Read the model definition and answer for the solid it produces. Units are mm, in the model's axes. A direction names the side the tool comes from. Round coordinates to 2 decimals unless told otherwise and drop trailing zeros. Write each loop counter-clockwise with the first axis right and the second up, starting at its lowest first coordinate (ties: lowest second). Pieces come first, ordered by that corner, then holes. Notation, with made-up numbers: (20, 70.25) -> (54, 70.25) arc R28 ccw to (54, 91.25) -> close; hole circle Ø8 at (-19.5, -8.5). An arc over 180 degrees is marked (long way). Return JSON: item names as keys, results as strings.
from build123d import *

# Parameters (mm, degrees)
SKETCH_1_R          = 7
SKETCH_1_R_2        = 1.5
EXTRUDE_1_DEPTH     = 14
FILLET_2_R          = 1
FILLET_4_R          = 2
FILLET_5_R          = 1
CUT_EXTRUDE_1_DEPTH = 10
FILLET_6_R          = 1
SKETCH_4_R          = 43
SKETCH_4_W          = 56
SKETCH_4_H          = 56
CUT_EXTRUDE_2_DEPTH = 2


with BuildPart() as part:
    # 草图1 → 凸台-拉伸1 (new body)
    # profile 1 of 3: a face of its own
    with BuildSketch(Plane.XY):
        with BuildLine():
            Line((-2.5, 7), (-20, 7))
            ThreePointArc((-20, 7), (-15.050252532, 4.949747468), (-13, 0))
            ThreePointArc((-13, 0), (-15.050252532, -4.949747468), (-20, -7))
            Line((-20, -7), (0, -7))
            ThreePointArc((0, -7), (-4.949747468, 4.949747468), (7, 0))
            Line((7, 0), (7, 4))
            Line((7, 4), (12, 4))
            Line((12, 4), (12, 5))
            Line((12, 5), (6.5, 9))
            Line((6.5, 9), (3.5, 9))
            Line((3.5, 9), (3.5, 26))
            Line((3.5, 26), (-2.5, 26))
            Line((-2.5, 26), (-2.5, 7))
        make_face()
    # profile 2 of 3: a face of its own
    with BuildSketch(Plane.XY):
        Circle(SKETCH_1_R)
        Circle(SKETCH_1_R_2, mode=Mode.SUBTRACT)
    # profile 3 of 3: a face of its own
    with BuildSketch(Plane.XY):
        with Locations((-20, 0)):
            Circle(SKETCH_1_R)
        with Locations((-20, 0)):
            Circle(SKETCH_1_R_2, mode=Mode.SUBTRACT)
    extrude(amount=EXTRUDE_1_DEPTH)

    # 圆角2
    fillet_2_edges = [part.edges().sort_by_distance(p)[0] for p in [
        (-2.5, 7, 7),
        (7, 4, 7),
    ]]
    fillet(fillet_2_edges, radius=FILLET_2_R)

    # 圆角4
    fillet_4_edges = [part.edges().sort_by_distance(p)[0] for p in [
        (6.5, 9, 7),
    ]]
    fillet(fillet_4_edges, radius=FILLET_4_R)

    # 圆角5
    fillet_5_edges = [part.edges().sort_by_distance(p)[0] for p in [
        (12, 5, 7),
    ]]
    fillet(fillet_5_edges, radius=FILLET_5_R)

    # 草图2 → 切除-拉伸1 (cut)
    with BuildSketch(Plane(origin=(3.5, 0, 0), x_dir=(0, 0, -1), z_dir=(1, 0, 0))):
        Polygon((-12, 9), (-14, 9), (-14, 26), (0, 26), (0, 9), (-2, 9), (-2, 24), (-12, 24), align=None)
    extrude(amount=-CUT_EXTRUDE_1_DEPTH, mode=Mode.SUBTRACT)

    # 圆角6
    fillet_6_edges = [part.edges().sort_by_distance(p)[0] for p in [
        (0.5, 24, 12),
        (0.5, 24, 2),
    ]]
    fillet(fillet_6_edges, radius=FILLET_6_R)

    # 草图4 → 切除-拉伸2 (cut)
    with BuildSketch(Plane.XY.offset(14)):
        with Locations((31.5, 37)):
            Circle(SKETCH_4_R)
        with Locations((31.5, 37)):
            Rectangle(SKETCH_4_W, SKETCH_4_H, mode=Mode.SUBTRACT)
    cut_extrude_2 = extrude(amount=-CUT_EXTRUDE_2_DEPTH, mode=Mode.SUBTRACT)

    # 镜向1: 切除-拉伸2 across plane
    add(cut_extrude_2.mirror(Plane.XY.offset(7)), mode=Mode.SUBTRACT)


solid = part.part
Item 1: For a pull along X with two mould halves and no side action, classify faces 1 (the flat face through (9.339, 6.935, 6.93)), 2 (the cylindrical face through (-1.5, 0.07, 6.9)), 3 (the flat face through (-10, -1, 0)) as released by +X, released by -X, zero draft, split by the parting line, or undercut.
Worked answers:
{"face 1": "released by +X", "face 2": "undercut", "face 3": "zero draft"}
Item 2: Section A-A (z = 10.25) is taken. Give the vertices of the cut face in (x, y), then the cut area to 3 significant figures.
Worked answers:
{"outline": "(-20, -7) -> (0, -7) arc R7 ccw to (7, 0) -> (7, 3) arc R1 cw to (8, 4) -> (12, 4) -> (12, 4.49) arc R1 ccw to (11.59, 5.3) -> (7.03, 8.62) arc R2 ccw to (5.85, 9) -> (3.5, 9) -> (3.5, 24) -> (-2.5, 24) -> (-2.5, 8) arc R1 cw to (-3.5, 7) -> (-20, 7) arc R7 ccw to start; hole circle Ø3 at (-20, 0); hole circle Ø3 at (0, 0)", "area": "554 mm2"}
Item 3: A tool of negligible diameter and unlimited length cuts with its end or side. For faces 4 (the flat face through (-2, 9, 13)), 5 (the flat face through (-2, 9, 1)), 6 (the cylindrical face through (2.641, 5.123, 0.986)), 7 (the flat face through (-2.5, 16, 7)), 8 (the flat face through (5, 9, 7)), from which of +Z, -Z, +X, -X, +Y, -Y can it reach the whole face along a straight path? Write none if from no direction.
Worked answers:
{"face 4": "+Z, +X, -X, +Y", "face 5": "-Z, +X, -X, +Y", "face 6": "-Z, +X, +Y", "face 7": "+Z, -Z, -X, +Y", "face 8": "+Z, -Z, +X, +Y"}
Item 4: Straight lines are drawn through the part: L1, parallel to Y at x = 0, z = 9.5; L2, parallel to Y at x = -20, z = 4.75; L3, parallel to Y at x = -3.5, z = 7. For each, find the intervals that lie inside material, in ascending order. Write a range as [from, to].
Worked answers:
{"L1": "y = [-7, -1.5], [1.5, 24]", "L2": "y = [-7, -1.5], [1.5, 7]", "L3": "y = [-7, 7]"}
Item 5: Section C-C (y = 10.5) is taken. Give the vertices of the cut face in (x, z).
Worked answers:
{"outline": "(-2.5, 2) -> (3.5, 2) -> (3.5, 12) -> (-2.5, 12) -> close"}
Item 6: Section B-B (x = 1) is taken. Give the vertices of the cut face in (y, z).
Worked answers:
{"outline": "(-6.93, 0) -> (-1.12, 0) -> (-1.12, 14) -> (-6.93, 14) -> close; (1.12, 0) -> (6.69, 0) -> (6.69, 2) -> (23, 2) arc R1 ccw to (24, 3) -> (24, 11) arc R1 ccw to (23, 12) -> (6.69, 12) -> (6.69, 14) -> (1.12, 14) -> close"}
Item 7: Flat-ended cylindrical pins translate along their axes: pin 1 (8 mm diameter, centred on x = 5, z = 7.5, fed in from -Y); pin 2 (4 mm diameter, centred on x = -23, z = 6, fed in from +Y); pin 3 (2.5 mm diameter, centred on x = -20, y = 0, fed in from +Z); pin 4 (0.7 mm diameter, centred on x = 4.5, z = 7, fed in from +Y). Find the tip coordinate at first contact, or state that the pin passes through.
Worked answers:
{"pin 1": "stops at y = -6.93", "pin 2": "stops at y = 6.93", "pin 3": "passes through", "pin 4": "stops at y = 9"}
Item 8: Section D-D (x = -15.5) is taken. Give the vertices of the cut face in (y, z).
Worked answers:
{"outline": "(-7, 0) -> (7, 0) -> (7, 14) -> (-7, 14) -> close"}
